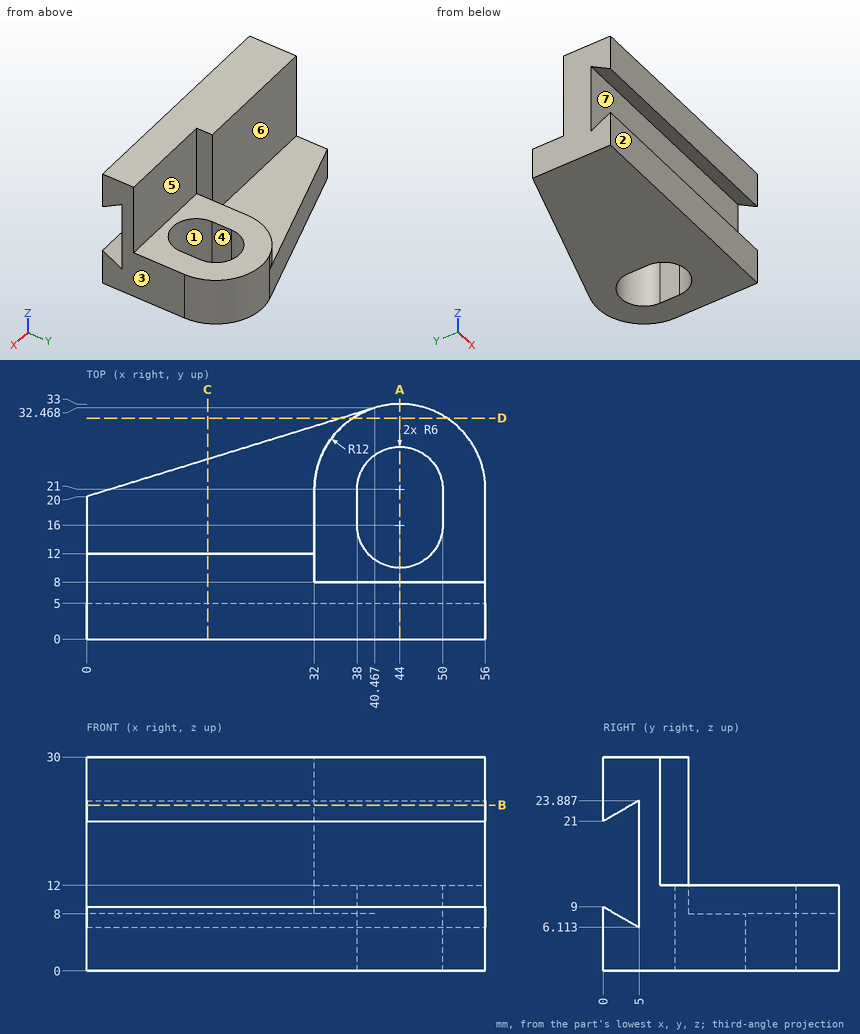
Print and shaded views of the part. All mm, measured from the part's lowest x, y and z. A direction names the side the tool comes from. Coordinates: 2 decimals unless noted, no trailing zeros. Order: outer loops, then holes, each group sorted by start corner. A loop starts at its lowest first (then second) coordinate and runs counter-clockwise, first axis right, second up. Notation, with made-up numbers: M 24.5,27.25 L 52.5,27.25 A20 ccw 52.5,62.25 Z; hole C -35,17 d9. An arc over 180 degrees is marked long. Write each question's results on one line, items separated by ' | '. Start each with the question number.
Q1. Cut at A-A (x = 44). List the corners of the cut face in (y, z).
Q2. Pull direction X, two halves, no side cores. Call the marked faces 1, 2 and 3: +X half, -X half, draft (parallel to the pull), parting line (faces both ways), or undercut.
Q3. Which spindle directions (+Z, -Z, +X, -X, +Y, -Y) get a long thin tool onto all of the face, cutting with end or side? Do the marked faces 4, 5, 6 and 7. Say none if no direction does.
Q4. Cut at D-D (y = 31). List the corners of the cut face in (x, z).
Q5. Cut at B-B (z = 23.25). List the corners of the cut face in (x, y), then the cut area to 3 significant figures.
Q6. Cut at C-C (x = 17). List the corners of the cut face in (y, z).
Q7. Flat gauge pins, fed straight in: P1, Ø1.2, axis at y = 15, z = 10.5, coming from the -X side; P2, Ø9, axis at x = 14.5, z = 15, coming from the -Y side; P3, Ø3, axis at x = 34.5, z = 7, coming from the +Y side. Where does each tip first touch, or does it go through?
Q8. Drill centre lines: probe 1 along X at (y, z) = (17.5, 7.5); probe 2 along X at (y, z) = (9, 27); probe 3 along Z at (x, y) = (41, 3.5). Where is each one in solid material? Low to high. Write a range as from..to.
Found:
1) outline: M 0,0 L 10,0 L 10,12 L 8,12 L 8,30 L 0,30 L 0,21 L 5,23.89 L 5,6.11 L 0,9 Z; M 27,0 L 33,0 L 33,12 L 27,12 Z
2) face 1: undercut | face 2: draft | face 3: +X half
3) face 4: +Z, -Z | face 5: +Z, +X, +Y | face 6: +Z, -X, +Y | face 7: +X, -X
4) outline: M 35.7,0 L 50.63,0 L 50.63,12 L 37.37,12 L 37.37,8 L 35.7,8 Z
5) outline: M 0,0 L 56,0 L 56,3.9 L 0,3.9 Z; M 0,5 L 56,5 L 56,8 L 32,8 L 32,12 L 0,12 Z | area: 514 mm²
6) outline: M 0,0 L 25.24,0 L 25.24,8 L 12,8 L 12,30 L 0,30 L 0,21 L 5,23.89 L 5,6.11 L 0,9 Z
7) P1: x = 32 | P2: y = 5 | P3: y = 31.09
8) probe 1: 0..38, 50..56 | probe 2: 0..32 | probe 3: 0..6.98, 23.02..30
